```python
from build123d import *

# Parameters (mm, degrees)
SKETCH1_W           = 14
SKETCH1_H           = 14
BOSS_EXTRUDE1_DEPTH = 45
SKETCH2_W           = 14
SKETCH2_H           = 4
BOSS_EXTRUDE2_DEPTH = 2.1


with BuildPart() as part:
    # Sketch1 → Boss-Extrude1 (new body)
    with BuildSketch(Plane(origin=(0, 0, 0), x_dir=(1, 0, 0), z_dir=(0, 1, 0))):
        with Locations((7, 7)):
            Rectangle(SKETCH1_W, SKETCH1_H)
    extrude(amount=BOSS_EXTRUDE1_DEPTH)

    # Sketch2 → Boss-Extrude2 (add)
    with BuildSketch(Plane(origin=(0, 0, -14), x_dir=(-1, 0, 0), z_dir=(0, 0, -1))):
        with Locations((-7, 37.706344583)):
            Rectangle(SKETCH2_W, SKETCH2_H)
        with Locations((-7, 12.706344583)):
            Rectangle(SKETCH2_W, SKETCH2_H)
    boss_extrude2 = extrude(amount=BOSS_EXTRUDE2_DEPTH)

    # Mirror1: Boss-Extrude2 across plane
    add(boss_extrude2.mirror(Plane.XY.offset(-7)))


solid = part.part
```
Geometry: final body of the model. Coordinates: model frame, mm. A direction names the side the tool comes from. Round coordinates to 2 decimals unless told otherwise and drop trailing zeros. Order: outer loops, then holes, each group sorted by start corner. A loop starts at its lowest first (then second) coordinate and runs counter-clockwise, first axis right, second up. Notation, with made-up numbers: (4, -32.75) -> (13, -32.75) arc R28 cw to (13, 2.25) -> close; hole circle Ø1 at (64.25, 43). An arc over 180 degrees is marked (long way). Use CSV: the item, a comma, the result in double quotes. Start each with the question number.
1) Section B-B (y = 25.5). Return the cut outline in (x, z), and give its area (3 significant figures).
2) First-contact query: pin 1 Ø1.1 at (x, z) = (5, -15.5) entering from -Y; pin 2 Ø2.5 at (x, z) = (9, 1.5) entering from +Y; pin 3 Ø1.6 at (x, y) = (5, 43) entering from -Z. Flat tips, straight axial feed; report the tip coordinate or a pass-through.
3) Material intervals for line 1 along Z through (x, y) = (4.25, 22.5); line 2 along Y through (x, z) = (9.5, 0.75), sorted ascending. Write a range as from..to.
4) Set-up query: faces 1 (the face through (7, 42, 0)), 2 (the face through (7, 25, 0)), 3 (the face through (7, 14.706, -15)), 4 (the face through (7, 42, -14)). Return all of +Z, -Z, +X, -X, +Y, -Y with unobstructed straight access to the full face (end or side cutting, diameter ignored); none if empty.
5) Draft query along Y for faces 5 (the face through (7, 38, 2.1)), 6 (the face through (7, 35.706, 1)), 7 (the face through (7, 10.706, 1)). Return one class per face: +Y half, -Y half, draft (parallel to the pull), parting line (faces both ways), or undercut.
6) Section A-A (x = 10.5). Return the cut outline in (y, z).
Returned:
1,outline,"(0, -14) -> (14, -14) -> (14, 0) -> (0, 0) -> close"
1,area,"196 mm²"
2,pin 1,"stops at y = 10.71"
2,pin 2,"stops at y = 39.71"
2,pin 3,"stops at z = -14"
3,line 1,"z = -14..0"
3,line 2,"y = 10.71..14.71, 35.71..39.71"
4,face 1,"+Z, +X, -X, +Y"
4,face 2,"+Z, +X, -X"
4,face 3,"-Z, +X, -X"
4,face 4,"-Z, +X, -X, +Y"
5,face 5,"draft"
5,face 6,"undercut"
5,face 7,"-Y half"
6,outline,"(0, -14) -> (10.71, -14) -> (10.71, -16.1) -> (14.71, -16.1) -> (14.71, -14) -> (35.71, -14) -> (35.71, -16.1) -> (39.71, -16.1) -> (39.71, -14) -> (45, -14) -> (45, 0) -> (39.71, 0) -> (39.71, 2.1) -> (35.71, 2.1) -> (35.71, 0) -> (14.71, 0) -> (14.71, 2.1) -> (10.71, 2.1) -> (10.71, 0) -> (0, 0) -> close"
